Job drawing, mm, ordinate dimensions from the low corner. One solid piece. Coordinates: 2 decimals unless noted, no trailing zeros. Loops run counter-clockwise (first coordinate to the right, second up) from the corner with the lowest first, then second, coordinate; pieces in that order, holes last. Notation, with made-up numbers: (-38, -10) -> (-34, -10) arc R20 cw to (-34, -1) -> close; hole circle Ø9 at (34, 29.25). An arc over 180 degrees is marked (long way). Use one line per item in the form item = value. Start each with the question number.
(1) Mould opens along X. For the marked faces 1 and 2 say: +X half, -X half, draft (parallel to the pull), parting line (faces both ways), or undercut.
(2) Pin check, flat tip, straight feed: P1, Ø6, axis at x = 64.5, z = 247.5, coming from the -Y side. Stop position of the tip, or through.
(3) Band-saw the part on D-D on x = 18. Give the cut face in (y, z).
(4) Drill centre lines: L1, parallel to X at y = 8, z = 213; L2, parallel to Y at x = 25, z = 256.5; L3, parallel to X at y = 14, z = 230.5. Where is each one in solid material? Low to high. Write a range as [from, to].
(5) Band-saw the part on B-B on y = 2.75. Give the cut face in (x, z).
(6) Band-saw the part on A-A on x = 38.1. Give the cut face in (y, z).
(7) Band-saw the part on C-C on z = 76. Give the cut face in (x, y).
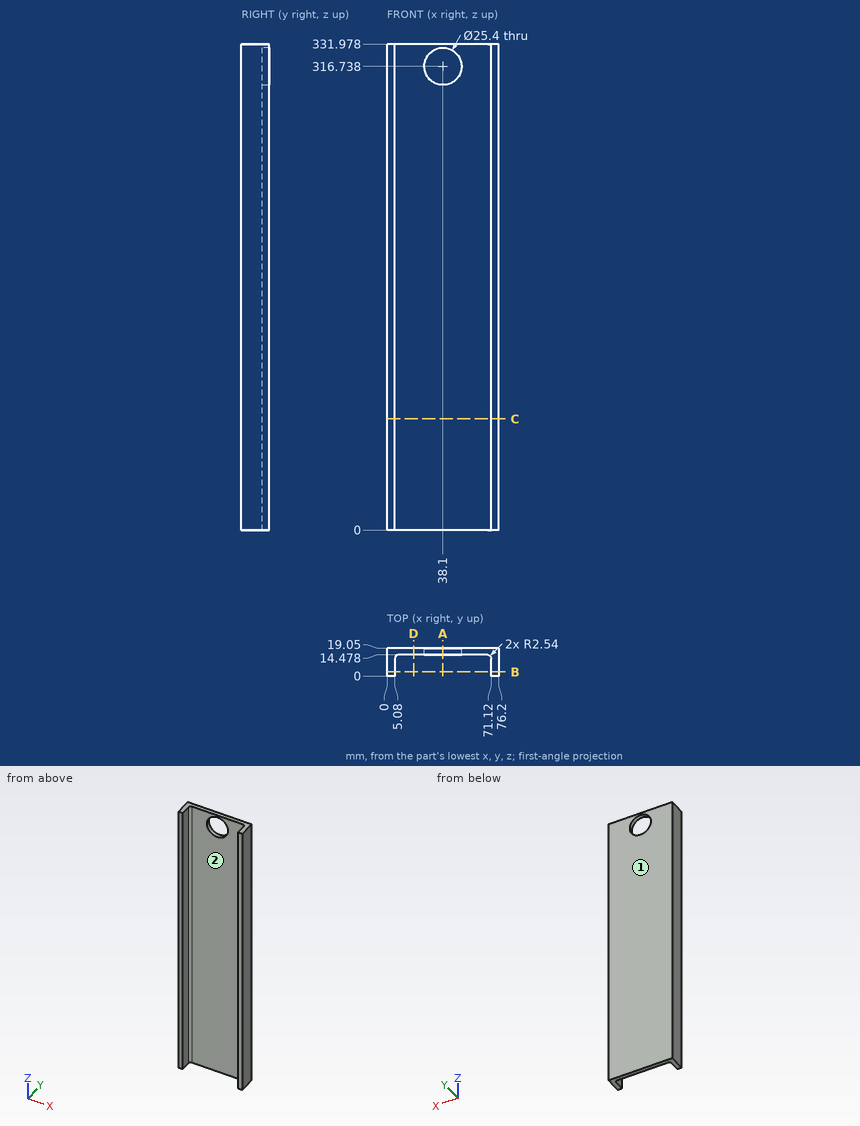
A:
q1.face_1 = draft
q1.face_2 = undercut
q2.P1 = 14.48
q3.outline = (14.48, 0) -> (19.05, 0) -> (19.05, 331.98) -> (14.48, 331.98) -> close
q4.L1 = [0, 5.08], [71.12, 76.2]
q4.L2 = [14.48, 19.05]
q4.L3 = [0, 6.14], [70.06, 76.2]
q5.outline = (0, 0) -> (5.08, 0) -> (5.08, 331.98) -> (0, 331.98) -> close; (71.12, 0) -> (76.2, 0) -> (76.2, 331.98) -> (71.12, 331.98) -> close
q6.outline = (14.48, 0) -> (19.05, 0) -> (19.05, 304.04) -> (14.48, 304.04) -> close; (14.48, 329.44) -> (19.05, 329.44) -> (19.05, 331.98) -> (14.48, 331.98) -> close
q7.outline = (0, 0) -> (5.08, 0) -> (5.08, 11.94) arc R2.54 cw to (7.62, 14.48) -> (68.58, 14.48) arc R2.54 cw to (71.12, 11.94) -> (71.12, 0) -> (76.2, 0) -> (76.2, 19.05) -> (0, 19.05) -> close
